Input: part model. Units: mm. Frame: model coordinates. Face numbers are marked on the shaded views. A direction names the side the tool comes from. Round coordinates to 2 decimals unless told otherwise and drop trailing zeros. Loops run counter-clockwise (first coordinate to the right, second up) from the corner with the lowest first, then second, coordinate; pieces in that order, holes last. Notation, with made-up numbers: (0, 66.5) - (27, 66.5) arc R10 ccw to (27, 70.5) - close; hole circle Ø11 at (-33.5, 35). An arc over 180 degrees is marked (long way). One line per question, with ' | ' between items. Start each with the question number.
Item 1: Set-up query: the marked faces 4, 5, 6, 7 and 8. Return all of +Z, -Z, +X, -X, +Y, -Y with unobstructed straight access to the full face (end or side cutting, diameter ignored); none if empty.
Item 2: Material intervals for line 1 along Y through (x, z) = (-6, -11.5); line 2 along Y through (x, z) = (8, -18), sorted ascending.
Item 3: Section C-C, the plane z = -21.5. Return loops of the section in (x, y).
Item 4: Section B-B, the plane y = 32.5. Return loops of the section in (x, z), plus the area to 3 significant figures.
Item 5: Section D-D, the plane z = -12.75. Give the number of separate pieces and of enclosed holes in the cut face, plus the area to 3 significant figures.
Item 6: Section A-A, the plane y = 54.5. Return loops of the section in (x, z), plus the area to 3 significant figures.
Item 7: First-contact query: pin 1 (1.5 mm diameter, centred on x = -16, z = -12, fed in from +Y); pin 2 (3 mm diameter, centred on x = 4, z = -13, fed in from -Y); pin 3 (1.3 mm diameter, centred on x = 0.5, z = -21, fed in from +Y); pin 4 (1.6 mm diameter, centred on x = 5.5, y = 40.5, fed in from +Z). Flat tips, straight axial feed; report the tip coordinate or a pass-through.
Item 8: Draft query along Z for the marked faces 1, 2 and 3. Return one class per face: pulls with the +Z half, pulls with the -Z half, needs draft (parallel to the pull), parting line crosses it, or undercut.
```python
from build123d import *

# Parameters (mm, degrees)
BOSS_EXTRUDE1_DEPTH    = 10.16
SKETCH2_W              = 8.900000000000002
SKETCH2_H              = 11.800000000000011
CUT_EXTRUDE1_DEPTH     = 2.5
SKETCH5_R              = 2.9999999999999996
CUT_EXTRUDE2_DEPTH     = 5.7
SKETCH7_W              = 1.2999999999999998
SKETCH7_H              = 0.8000000000000007
SKETCH7_H_2            = 0.7999999999999936
BOSS_EXTRUDE2_DEPTH    = 4.5
CUT_EXTRUDE5_START     = -10.96
CUT_EXTRUDE5_DEPTH     = 10.96
SKETCH10_R             = 1.4999999999999998
CUT_EXTRUDE6_DEPTH     = 4.5
SKETCH13_W             = 3.75
SKETCH13_H             = 1
CUT_EXTRUDE8_DEPTH     = 3
FILLET3_R              = 0.5
FILLET4_R              = 1
SKETCH12_W             = 1.2999999999999998
SKETCH12_H             = 1.299999999999999
BOSS_EXTRUDE3_DEPTH    = 0.5
BOSS_EXTRUDE3_2_DEPTH  = 0.5
BOSS_EXTRUDE3_3_DEPTH  = 0.5
BOSS_EXTRUDE4_START    = 0.01
BOSS_EXTRUDE4_DEPTH    = 0.01
LPATTERN8_COUNT        = 3
LPATTERN8_PITCH        = 10.16
LPATTERN8_2_COUNT      = 3
LPATTERN8_2_PITCH      = 10.16
LPATTERN8_3_COUNT      = 3
LPATTERN8_3_PITCH      = 10.16
LPATTERN8_4_COUNT      = 3
LPATTERN8_4_PITCH      = 10.16
FILLET3_OF_LPATTERN8_R = 0.5
FILLET4_OF_LPATTERN8_R = 1
SKETCH11_W             = 1.6
SKETCH11_H             = 8
CUT_EXTRUDE7_DEPTH     = 1.5
LPATTERN9_COUNT        = 2
LPATTERN9_PITCH        = 10.16
BOSS_EXTRUDE6_DEPTH    = 0.01


# Read off the part's stored shape, not the designer's step: Cut-Extrude5
with BuildPart() as part:
    # Sketch1 → Boss-Extrude1 (new body)
    with BuildSketch(Plane(origin=(0, 0, 0), x_dir=(0, 0, -1), z_dir=(1, 0, 0))):
        Polygon((9.669213470381848, 32.96915259715871), (9.669213470381848, 47.08678337249189), (13.847501539912686, 47.08678337249189), (14.859335014289963, 58.54185616450892), (26.70903057031256, 58.54185616450892), (28.514863984729242, 47.38649061080074), (29.669213470381848, 47.38649061080074), (29.66921347038185, 29.041856164508925), (11.142277404209432, 29.04185616450892), (11.142277404209432, 32.96915259715871), align=None)
    boss_extrude1 = extrude(amount=BOSS_EXTRUDE1_DEPTH)

    # Sketch2 → Cut-Extrude1 (cut)
    with BuildSketch(Plane.XY.offset(-9.669213470381848)):
        with Locations((5.08, 40.0279679848253)):
            Rectangle(SKETCH2_W, SKETCH2_H)
    cut_extrude1 = extrude(amount=-CUT_EXTRUDE1_DEPTH, mode=Mode.SUBTRACT)

    # Sketch3 → Cut-Loft1 section 0
    with BuildSketch(Plane.XY.offset(-12.169213470381848)):
        with BuildLine():
            Line((9.530000000000001, 34.1279679848253), (9.530000000000001, 45.92796798482531))
            Line((9.530000000000001, 45.92796798482531), (0.6299999999999994, 45.92796798482531))
            Line((0.6299999999999994, 45.92796798482531), (0.6299999999999994, 34.1279679848253))
            Line((0.6299999999999994, 34.1279679848253), (9.530000000000001, 34.1279679848253))
        make_face()
    # Sketch4 → Cut-Loft1 section 1
    with BuildSketch(Plane.XY.offset(-14.069213470381849)):
        with BuildLine():
            Line((2.3299999999999987, 36.877967984825304), (7.829999999999998, 36.877967984825304))
            Line((7.829999999999998, 36.877967984825304), (7.829999999999998, 43.1779679848253))
            Line((7.829999999999998, 43.1779679848253), (2.3299999999999987, 43.1779679848253))
            Line((2.3299999999999987, 43.1779679848253), (2.3299999999999987, 36.877967984825304))
        make_face()
    cut_loft1 = loft(mode=Mode.SUBTRACT)

    # Sketch5 → Cut-Extrude2 (cut)
    with BuildSketch(Plane(origin=(0, 58.54185616450892, 0), x_dir=(1, 0, 0), z_dir=(0, 1, 0))):
        with Locations(Location((5.08, 20.784182792301262, 0), (0, 0, 270))):
            Circle(SKETCH5_R)
    cut_extrude2 = extrude(amount=-CUT_EXTRUDE2_DEPTH, mode=Mode.SUBTRACT)

    # Sketch7 → Boss-Extrude2 (add)
    with BuildSketch(Plane.XZ.offset(-29.041856164508918)):
        with Locations((5.08, -27.169213470381862)):
            Rectangle(SKETCH7_W, SKETCH7_H)
        with Locations((5.08, -17.00921347038186)):
            Rectangle(SKETCH7_W, SKETCH7_H_2)
    boss_extrude2 = extrude(amount=BOSS_EXTRUDE2_DEPTH)

    # Cut-Extrude5 outline → Cut-Extrude5 (cut)
    with BuildSketch(Plane.XY.offset(-16.60921347038186).offset(CUT_EXTRUDE5_START)):
        with BuildLine():
            Line((5.73, 24.541856165), (5.73, 25.191856165))
            ThreePointArc((5.73, 25.191856165), (5.539619408, 24.732236757), (5.08, 24.541856165))
            Line((5.08, 24.541856165), (5.73, 24.541856165))
        make_face()
        with BuildLine():
            Line((4.43, 24.541856165), (5.08, 24.541856165))
            ThreePointArc((5.08, 24.541856165), (4.620380592, 24.732236757), (4.43, 25.191856165))
            Line((4.43, 25.191856165), (4.43, 24.541856165))
        make_face()
    cut_extrude5 = extrude(amount=CUT_EXTRUDE5_DEPTH, mode=Mode.SUBTRACT)

    # Sketch10 → Cut-Extrude6 (cut)
    with BuildSketch(Plane(origin=(0, 38.527852040591384, -38.527852040591256), x_dir=(-1, 0, 0), z_dir=(0, 0.7071067811865488, -0.7071067811865464))):
        with Locations(Location((-5.08, 12.528006810151506, 0), (0, 0, 90))):
            Circle(SKETCH10_R)
    cut_extrude6 = extrude(amount=-CUT_EXTRUDE6_DEPTH, mode=Mode.SUBTRACT)

    # Sketch13 → Cut-Extrude8 (cut)
    with BuildSketch(Plane.XY.offset(-11.142277404209432)):
        with Locations((5.080000000000007, 31.005504380833823)):
            Rectangle(SKETCH13_W, SKETCH13_H)
    cut_extrude8 = extrude(amount=-CUT_EXTRUDE8_DEPTH, mode=Mode.SUBTRACT)

    # Fillet3
    fillet3_edges = [part.edges().sort_by_distance(p)[0] for p in [
        (5.08, 58.54185616450892, -26.70903057031256),
    ]]
    fillet(fillet3_edges, radius=FILLET3_R)

    # Fillet4
    fillet4_edges = [part.edges().sort_by_distance(p)[0] for p in [
        (5.08, 58.54185616450892, -14.859335014289963),
    ]]
    fillet(fillet4_edges, radius=FILLET4_R)

    # Sketch14 → Boss-Extrude4 (add)
    with BuildSketch(Plane(origin=(10.16, 0, 0), x_dir=(0, 0, -1), z_dir=(1, 0, 0)).offset(BOSS_EXTRUDE4_START)):
        with BuildLine():
            Line((14.77877644669124, 57.629844179105966), (13.847501539912686, 47.08678337249189))
            Line((13.847501539912686, 47.08678337249189), (9.669213470381848, 47.08678337249189))
            Line((9.669213470381848, 47.08678337249189), (9.669213470381848, 32.96915259715871))
            Line((9.669213470381848, 32.96915259715871), (11.142277404209432, 32.96915259715871))
            Line((11.142277404209432, 32.96915259715871), (11.142277404209432, 29.04185616450892))
            Line((11.142277404209432, 29.04185616450892), (29.66921347038185, 29.041856164508925))
            Line((29.66921347038185, 29.041856164508925), (29.669213470381848, 47.38649061080074))
            Line((29.669213470381848, 47.38649061080074), (28.514863984729242, 47.38649061080074))
            Line((28.514863984729242, 47.38649061080074), (26.777036465378647, 58.121756163471794))
            ThreePointArc((26.777036465378647, 58.121756163471794), (26.607537368480997, 58.42261199143836), (26.28346175961899, 58.54185616450892))
            Line((26.28346175961899, 58.54185616450892), (15.77489798008326, 58.54185616450892))
            ThreePointArc((15.77489798008326, 58.54185616450892), (15.09961582223998, 58.279415658582806), (14.77877644669124, 57.629844179105966))
        make_face()
    extrude(amount=-BOSS_EXTRUDE4_DEPTH)



with BuildPart() as body_2:
    # Sketch12 → Boss-Extrude3 (new body)
    with BuildSketch(Plane.XZ.offset(-29.041856164508918)):
        with Locations((3.9e-16, -15.192277404209438)):
            Rectangle(SKETCH12_W, SKETCH12_H)
    boss_extrude3 = extrude(amount=BOSS_EXTRUDE3_DEPTH)


with BuildPart() as body_3:
    # Sketch12 → Boss-Extrude3 2 (new body)
    with BuildSketch(Plane.XZ.offset(-29.041856164508918)):
        Polygon((-0.6500000000000012, -20.342277404209444), (0.6499999999999989, -20.342277404209444), (0.649999999999998, -19.04227740420944), (-0.6500000000000012, -19.04227740420944), align=None)
    boss_extrude3_2 = extrude(amount=BOSS_EXTRUDE3_2_DEPTH)


with BuildPart() as body_4:
    # Sketch12 → Boss-Extrude3 3 (new body)
    with BuildSketch(Plane.XZ.offset(-29.041856164508918)):
        Polygon((-0.6499999999999996, -25.042277404209447), (0.6500000000000006, -25.042277404209447), (0.6500000000000008, -23.742277404209442), (-0.6499999999999996, -23.742277404209442), align=None)
    boss_extrude3_3 = extrude(amount=BOSS_EXTRUDE3_3_DEPTH)


with BuildPart() as part_1:
    add(part.part)

    add(body_2.part)  # LPattern8 merges body 2

    add(body_3.part)  # LPattern8 merges body 3

    add(body_4.part)  # LPattern8 merges body 4
    # LPattern8: Boss-Extrude1 ×3
    with Locations(*[(-i * LPATTERN8_PITCH, 0, 0) for i in range(1, LPATTERN8_COUNT)]):
        add(boss_extrude1)

    # LPattern8 2: Cut-Extrude1, Cut-Loft1, Cut-Extrude2 ×3
    with Locations(*[(-i * LPATTERN8_2_PITCH, 0, 0) for i in range(1, LPATTERN8_2_COUNT)]):
        add(cut_extrude1, mode=Mode.SUBTRACT)
        add(cut_loft1, mode=Mode.SUBTRACT)
        add(cut_extrude2, mode=Mode.SUBTRACT)

    # LPattern8 3: Boss-Extrude2 ×3
    with Locations(*[(-i * LPATTERN8_3_PITCH, 0, 0) for i in range(1, LPATTERN8_3_COUNT)]):
        add(boss_extrude2)

    # LPattern8 4: Cut-Extrude5, Cut-Extrude6, Cut-Extrude8 ×3
    with Locations(*[(-i * LPATTERN8_4_PITCH, 0, 0) for i in range(1, LPATTERN8_4_COUNT)]):
        add(cut_extrude5, mode=Mode.SUBTRACT)
        add(cut_extrude6, mode=Mode.SUBTRACT)
        add(cut_extrude8, mode=Mode.SUBTRACT)

    # Fillet3 of LPattern8
    fillet3_of_lpattern8_edges = [part_1.edges().sort_by_distance(p)[0] for p in [
        (-5.08, 58.54185616450892, -26.70903057031256),
        (-15.24, 58.54185616450892, -26.70903057031256),
    ]]
    fillet(fillet3_of_lpattern8_edges, radius=FILLET3_OF_LPATTERN8_R)

    # Fillet4 of LPattern8
    fillet4_of_lpattern8_edges = [part_1.edges().sort_by_distance(p)[0] for p in [
        (-5.08, 58.54185616450892, -14.859335014289963),
        (-15.24, 58.54185616450892, -14.859335014289963),
    ]]
    fillet(fillet4_of_lpattern8_edges, radius=FILLET4_OF_LPATTERN8_R)

    # Sketch11 → Cut-Extrude7 (cut)
    with BuildSketch(Plane(origin=(0, 58.54185616450892, 0), x_dir=(1, 0, 0), z_dir=(0, 1, 0))):
        with Locations((4.16e-15, 21.064117563348077)):
            Rectangle(SKETCH11_W, SKETCH11_H)
    cut_extrude7 = extrude(amount=-CUT_EXTRUDE7_DEPTH, mode=Mode.SUBTRACT)

    # LPattern9: Boss-Extrude3, Boss-Extrude3 2, Boss-Extrude3 3, Cut-Extrude7 ×2
    with Locations(*[(-i * LPATTERN9_PITCH, 0, 0) for i in range(1, LPATTERN9_COUNT)]):
        add(boss_extrude3)
        add(boss_extrude3_2)
        add(boss_extrude3_3)
        add(cut_extrude7, mode=Mode.SUBTRACT)

    # Sketch16 → Boss-Extrude6 (add)
    with BuildSketch(Plane.ZY.offset(20.32)):
        with BuildLine():
            Line((-13.847501539912686, 47.08678337249189), (-14.77877644669124, 57.629844179105966))
            ThreePointArc((-14.77877644669124, 57.629844179105966), (-15.09961582223998, 58.279415658582806), (-15.77489798008326, 58.54185616450892))
            Line((-15.77489798008326, 58.54185616450892), (-26.28346175961899, 58.54185616450892))
            ThreePointArc((-26.28346175961899, 58.54185616450892), (-26.607537368480997, 58.42261199143836), (-26.777036465378647, 58.121756163471794))
            Line((-26.777036465378647, 58.121756163471794), (-28.514863984729242, 47.38649061080074))
            Line((-28.514863984729242, 47.38649061080074), (-29.669213470381848, 47.38649061080074))
            Line((-29.669213470381848, 47.38649061080074), (-29.66921347038185, 29.041856164508925))
            Line((-29.66921347038185, 29.041856164508925), (-11.142277404209432, 29.04185616450892))
            Line((-11.142277404209432, 29.04185616450892), (-11.142277404209432, 32.96915259715871))
            Line((-11.142277404209432, 32.96915259715871), (-9.669213470381848, 32.96915259715871))
            Line((-9.669213470381848, 32.96915259715871), (-9.669213470381848, 47.08678337249189))
            Line((-9.669213470381848, 47.08678337249189), (-13.847501539912686, 47.08678337249189))
        make_face()
    extrude(amount=BOSS_EXTRUDE6_DEPTH)


solid = part_1.part
```
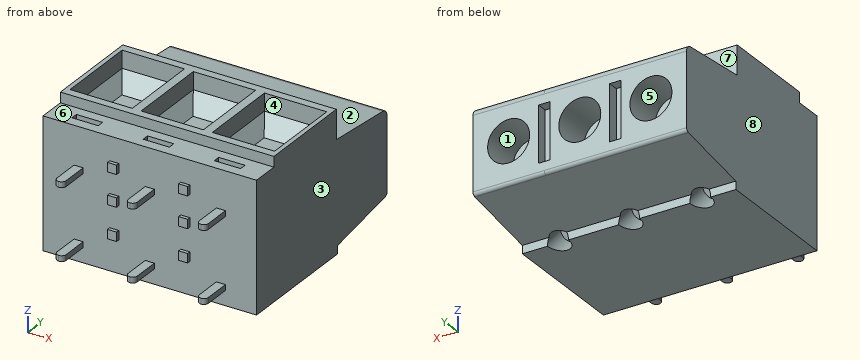
Return value:
1) face 4: +Z | face 5: +Y | face 6: +Z, +X, -X, -Y | face 7: +Z, +X, -X, +Y | face 8: +Z, -Z, -X, +Y, -Y
2) line 1: 29.04 to 30.51, 31.51 to 34.13, 45.93 to 47.09 | line 2: 29.04 to 58.54
3) outline: (-20.33, 29.04) - (10.17, 29.04) - (10.17, 58.54) - (7.99, 58.54) - (7.99, 52.84) - (2.17, 52.84) - (2.17, 58.54) - (0.8, 58.54) - (0.8, 57.04) - (-0.8, 57.04) - (-0.8, 58.54) - (-2.17, 58.54) - (-2.17, 52.84) - (-7.99, 52.84) - (-7.99, 58.54) - (-9.36, 58.54) - (-9.36, 57.04) - (-10.96, 57.04) - (-10.96, 58.54) - (-12.33, 58.54) - (-12.33, 52.84) - (-18.15, 52.84) - (-18.15, 58.54) - (-20.33, 58.54) - close
4) outline: (-20.33, -29.67) - (10.17, -29.67) - (10.17, -11.14) - (-20.33, -11.14) - close | area: 565 mm2
5) separate pieces: 1 | enclosed holes: 6 | area: 300 mm2
6) outline: (-20.33, -27.36) - (10.17, -27.36) - (10.17, -14.5) - (-20.33, -14.5) - close; hole circle Ø6 at (-15.24, -20.78); hole circle Ø6 at (-5.08, -20.78); hole circle Ø6 at (5.08, -20.78) | area: 307 mm2
7) pin 1: y = 47.09 | pin 2: y = 29.04 | pin 3: y = 58.54 | pin 4: z = -14.07
8) face 1: undercut | face 2: pulls with the +Z half | face 3: needs draft
